Can you work these out from the drawing? Everything is in mm from the part's minimum corner. A direction names the side the tool comes from. Round coordinates to 2 decimals unless told otherwise and drop trailing zeros. Loops run counter-clockwise (first coordinate to the right, second up) from the corner with the lowest first, then second, coordinate; pieces in that order, holes last. Notation, with made-up numbers: (-29, 53.25) - (28, 53.25) arc R12 cw to (28, 59.25) - close; hole circle Ø6 at (-7.75, 17). An arc over 180 degrees is marked (long way). Answer as a JSON object with one key per item and string values. Group by question number.
1) I want a section at D-D, the plane x = 4.1. Please give me the cut outline in (y, z).
2) Will this pin go through, and if not, where does the flat tip stop? P1, Ø1.6, axis at x = 3, y = 3, coming from the +Z side.
3) I want a section at C-C, the plane z = 3.6. Please give me the cut outline in (x, y).
4) I want a section at A-A, the plane x = 3. Please give me the cut outline in (y, z), then the cut area to 3 significant figures.
5) If I drill on line 1 along X through (y, z) = (3.05, 2.35); line 2 along X through (y, z) = (1.6, 0.3), over which ranges is the centre line in solid material (lowest first)? Write a range as [from, to].
6) I want a section at B-B, the plane y = 2.4. Please give me the cut outline in (x, z).
7) Which directions (+Z, -Z, +X, -X, +Y, -Y) give clear straight access to the entire face, cutting with the end or side of a thin tool? Please do the marked faces 1 and 2.
8) If we mould it in two halves opening along Y, with no side actions, what happens to the marked faces 3, 4, 5 and 6? For each: pulls with the +Y half, pulls with the -Y half, needs draft (parallel to the pull), parting line crosses it, or undercut.
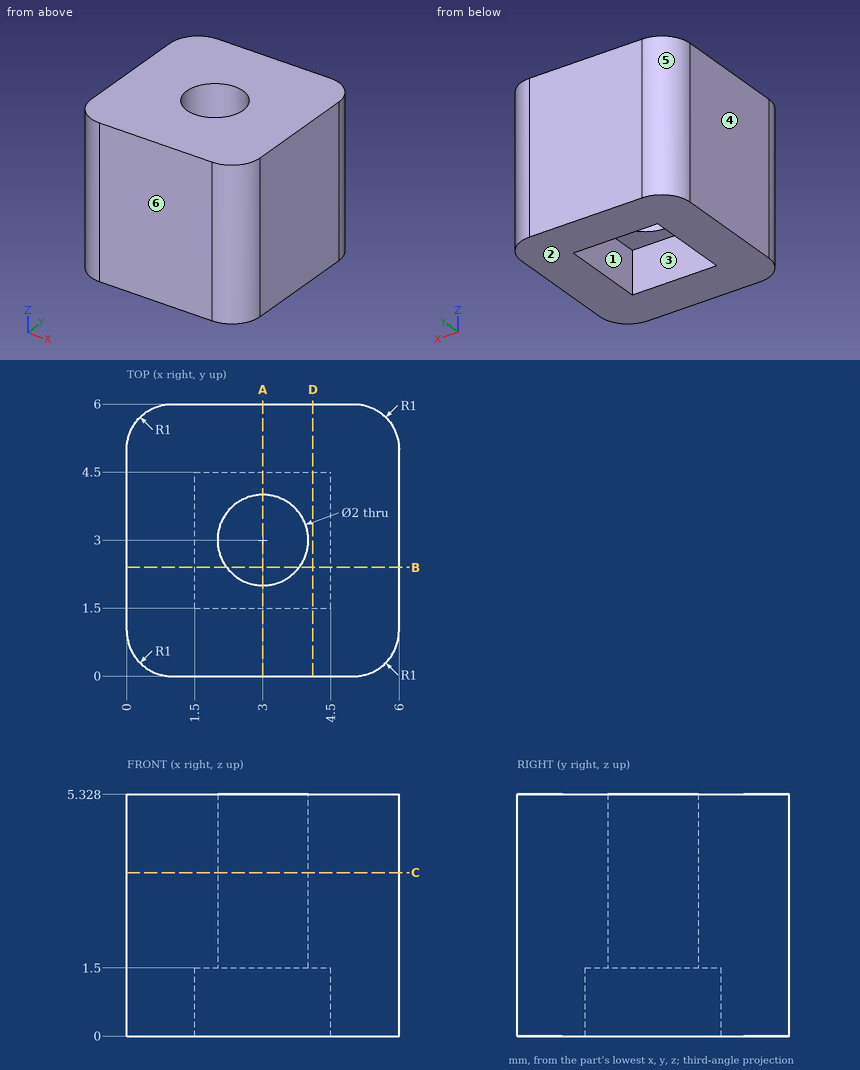
Outcome:
{
 "1": {"outline": "(0, 0) - (1.5, 0) - (1.5, 1.5) - (4.5, 1.5) - (4.5, 0) - (6, 0) - (6, 5.33) - (0, 5.33) - close"},
 "2": {"P1": "through"},
 "3": {"outline": "(0, 1) arc R1 ccw to (1, 0) - (5, 0) arc R1 ccw to (6, 1) - (6, 5) arc R1 ccw to (5, 6) - (1, 6) arc R1 ccw to (0, 5) - close; hole circle Ø2 at (3, 3)"},
 "4": {"outline": "(0, 0) - (1.5, 0) - (1.5, 1.5) - (2, 1.5) - (2, 5.33) - (0, 5.33) - close; (4, 1.5) - (4.5, 1.5) - (4.5, 0) - (6, 0) - (6, 5.33) - (4, 5.33) - close", "area": "19.8 mm^2"},
 "5": {"line 1": "[0, 2], [4, 6]", "line 2": "[0, 1.5], [4.5, 6]"},
 "6": {"outline": "(0, 0) - (1.5, 0) - (1.5, 1.5) - (2.2, 1.5) - (2.2, 5.33) - (0, 5.33) - close; (3.8, 1.5) - (4.5, 1.5) - (4.5, 0) - (6, 0) - (6, 5.33) - (3.8, 5.33) - close"},
 "7": {"face 1": "-Z", "face 2": "-Z, +X, -X, +Y, -Y"},
 "8": {"face 3": "undercut", "face 4": "needs draft", "face 5": "pulls with the +Y half", "face 6": "pulls with the -Y half"}
}
